Geometry check sheet. Reference: the model listing, model coordinates, mm. Round coordinates to 2 decimals unless told otherwise and drop trailing zeros. Use a Markdown table: item, result.
```python
from build123d import *

# Parameters (mm, degrees)
SKETCH1_W           = 378.46
SKETCH1_H           = 50.8
SKETCH1_R           = 2.032
BOSS_EXTRUDE1_DEPTH = 3.175
SKETCH2_R           = 12.7
CUT_EXTRUDE1_DEPTH  = 191.953485239
SKETCH3_R           = 2.032
CUT_EXTRUDE2_DEPTH  = 191.953485239
SKETCH4_R           = 2.032
CUT_EXTRUDE3_DEPTH  = 191.953485239
SKETCH6_R           = 2.032
CUT_EXTRUDE5_DEPTH  = 191.953485239
CUT_EXTRUDE6_DEPTH  = 191.953485239
FILLET1_R           = 12.7


with BuildPart() as part:
    # Sketch1 → Boss-Extrude1 (new body)
    with BuildSketch(Plane.XY):
        Rectangle(SKETCH1_W, SKETCH1_H)
        Circle(SKETCH1_R, mode=Mode.SUBTRACT)
        with Locations((-38.1, 0)):
            Circle(SKETCH1_R, mode=Mode.SUBTRACT)
        with Locations((-76.2, 0)):
            Circle(SKETCH1_R, mode=Mode.SUBTRACT)
        with Locations((-114.3, 0)):
            Circle(SKETCH1_R, mode=Mode.SUBTRACT)
        with Locations((-152.4, 0)):
            Circle(SKETCH1_R, mode=Mode.SUBTRACT)
        with Locations(Location((76.2, 0, 0), (0, 0, 180))):
            Circle(SKETCH1_R, mode=Mode.SUBTRACT)
        with Locations(Location((114.3, 0, 0), (0, 0, 180))):
            Circle(SKETCH1_R, mode=Mode.SUBTRACT)
        with Locations(Location((152.4, 0, 0), (0, 0, 180))):
            Circle(SKETCH1_R, mode=Mode.SUBTRACT)
        with Locations(Location((38.1, 0, 0), (0, 0, 180))):
            Circle(SKETCH1_R, mode=Mode.SUBTRACT)
    extrude(amount=BOSS_EXTRUDE1_DEPTH)

    # Sketch2 → Cut-Extrude1 (cut, through all)
    with BuildSketch(Plane.XY.offset(3.175)):
        Circle(SKETCH2_R)
    extrude(amount=-CUT_EXTRUDE1_DEPTH, mode=Mode.SUBTRACT)

    # Sketch3 → Cut-Extrude2 (cut, through all)
    with BuildSketch(Plane.XY.offset(3.175)):
        with Locations((-38.1, -19.05)):
            Circle(SKETCH3_R)
        with Locations((-44.45, 19.05)):
            Circle(SKETCH3_R)
        with Locations((44.45, 19.05)):
            Circle(SKETCH3_R)
        with Locations((38.1, -19.05)):
            Circle(SKETCH3_R)
    extrude(amount=-CUT_EXTRUDE2_DEPTH, mode=Mode.SUBTRACT)

    # Sketch4 → Cut-Extrude3 (cut, through all)
    with BuildSketch(Plane.XY.offset(3.175)):
        with Locations((-107.95, -19.05)):
            Circle(SKETCH4_R)
        with Locations((-120.65, -19.05)):
            Circle(SKETCH4_R)
        with Locations((-120.65, 19.05)):
            Circle(SKETCH4_R)
        with Locations((-107.95, 19.05)):
            Circle(SKETCH4_R)
    cut_extrude3 = extrude(amount=-CUT_EXTRUDE3_DEPTH, mode=Mode.SUBTRACT)

    # Sketch6 → Cut-Extrude5 (cut, through all)
    with BuildSketch(Plane.XY.offset(3.175)):
        with Locations((-182.88, 19.05)):
            Circle(SKETCH6_R)
        with Locations((-182.88, -19.05)):
            Circle(SKETCH6_R)
    cut_extrude5 = extrude(amount=-CUT_EXTRUDE5_DEPTH, mode=Mode.SUBTRACT)

    # Mirror1: Cut-Extrude3, Cut-Extrude5 across plane
    add(cut_extrude3.mirror(Plane(origin=(0, 0, 0), x_dir=(0, 0, 1), z_dir=(1, 0, 0))), mode=Mode.SUBTRACT)
    add(cut_extrude5.mirror(Plane(origin=(0, 0, 0), x_dir=(0, 0, 1), z_dir=(1, 0, 0))), mode=Mode.SUBTRACT)

    # Sketch7 → Cut-Extrude6 (cut, through all)
    with BuildSketch(Plane.XY.offset(3.175)):
        Polygon((-189.23, 0), (-163.83, -25.4), (-189.23, -25.4), align=None)
        Polygon((189.23, -25.4), (189.23, 0), (163.83, -25.4), align=None)
    extrude(amount=-CUT_EXTRUDE6_DEPTH, mode=Mode.SUBTRACT)

    # Fillet1
    fillet1_edges = [part.edges().sort_by_distance(p)[0] for p in [
        (-189.23, 0, 1.5875),
        (-163.83, -25.4, 1.5875),
        (163.83, -25.4, 1.5875),
        (189.23, 0, 1.5875),
    ]]
    fillet(fillet1_edges, radius=FILLET1_R)


solid = part.part
```
(1) Section check A-A on z = 1.4. State how many separate pieces and enclosed holes the cut face has, plus the area to 3 significant figures.
A:
| item | result |
|---|---|
| separate pieces | 1 |
| enclosed holes | 23 |
| area | 17,800 mm2 |
(2) Release check for a two-part mould opening along X. For faces 1 (the face through (-2.75, -12.4, 1.61)), 2 (the face through (-3, 17, 0)), 3 (the face through (-176.66, -12.57, 1.61)) record: +X half, -X half, draft (parallel to the pull), parting line (faces both ways), or undercut.
A:
| item | result |
|---|---|
| face 1 | undercut |
| face 2 | draft |
| face 3 | -X half |
(3) Thickness scan on line 1 (Y direction, x = 0, z = 1.55); line 2 (Y direction, x = -114.3, z = 1.15); line 3 (X direction, y = 4, z = 1.3). Record the ranges inside material, lowest first.
A:
| item | result |
|---|---|
| line 1 | y = -25.4 to -12.7, 12.7 to 25.4 |
| line 2 | y = -25.4 to -2.03, 2.03 to 25.4 |
| line 3 | x = -189.17 to -12.05, 12.05 to 189.17 |
